Check sheet for the modelled part. Datum: model origin and axes. Units: mm. Face numbers are marked on the shaded views. Give positions to 0.01 mm unless a question says otherwise; leave off trailing zeros. Order: outer loops, then holes, each group sorted by start corner. A loop starts at its lowest first (then second) coordinate and runs counter-clockwise, first axis right, second up.
Autodesk Inventor part; units mm, degrees
ref_plane "YZ Plane" through (0, 0, 0) normal (1, 0, 0) x (0, 1, 0)
ref_plane "XZ Plane" through (0, 0, 0) normal (0, 1, 0) x (-1, 0, 0)
ref_plane "XY Plane" through (0, 0, 0) normal (0, 0, 1) x (1, 0, 0)
sketch "Sketch1" plane through (0, 0, 0) normal (0, 1, 0) x (-1, 0, 0)
  circle A0 centre (0, 0) radius 1.9
  dimension "d0" = 3.8
extrude "Extrusion1" add sketch "Sketch1" along normal blind 6.2
sketch "Sketch2" plane through (0, 6.2, 0) normal (0, 1, 0) x (1, 0, 0)
  line L0 (0, 0) -> (0, -38.1) construction
  line L1 (-4, 0) -> (-4, -38.1)
  line L2 (4, -38.1) -> (4, 0)
  arc A0 (4, 0) -> (-4, 0) centre (0, 0) ccw
  line L3 (4, -38.1) -> (-4, -38.1)
  point P0 (0, -19.05)
  dimension "d6" = 4
  dimension "d7" = 38.1
extrude "Extrusion2" add sketch "Sketch2" along normal blind 0.75 and the other way blind 1.25
sketch "Sketch3" plane through (0, 4.95, 0) normal (0, -1, 0) x (1, 0, 0)
  circle A0 centre (0, 30.48) radius 1.5
  circle A1 centre (0, 0) radius 1.9
  dimension "d11" = 3
  dimension "d12" = 30.48
extrude "Extrusion3" cut sketch "Sketch3" against normal blind 1 contours A0
fillet "Fillet1" radius 1 2 edges at (-4, 5.95, 38.1) (4, 5.95, 38.1)
sketch "Sketch4" plane through (0, 0, 0) normal (0, -1, 0) x (1, 0, 0)
  circle A0 centre (0, 0) radius 1.1
  dimension "d18" = 2.2
extrude "Extrusion4" cut sketch "Sketch4" against normal blind 6.8
properties part number "CC-topHand" material "ABS Plastic"
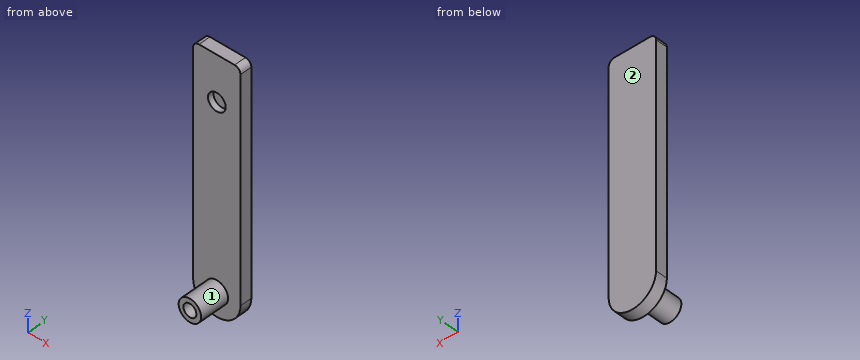
(1) Release check for a two-part mould opening along Z. For the marked faces 1 and 2 record: released by +Z, released by -Z, zero draft, split by the parting line, or undercut.
Response values:
face 1: split by the parting line
face 2: zero draft
(2) Material ranges on L1, parallel to Z at x = 0, y = 5.45; L2, parallel to Y at x = 0.75, z = 4; L3, parallel to X at y = 5.5, z = 1, recorded low to high.
Response values:
L1: z = -4 to -1.1, 1.1 to 28.98, 31.98 to 38.1
L2: y = 4.95 to 6.95
L3: x = -4 to -0.46, 0.46 to 4
(3) Cross-section at C-C on y = 4. Enter the section's corners in (x, z).
Response values:
outline: circle Ø3.8 at (0, 0); hole circle Ø2.2 at (0, 0)
(4) Cross-section at B-B on x = 0. Enter the section's corners in (y, z).
Response values:
outline: (0, -1.9) - (4.95, -1.9) - (4.95, -4) - (6.95, -4) - (6.95, 38.1) - (4.95, 38.1) - (4.95, 31.98) - (5.95, 31.98) - (5.95, 28.98) - (4.95, 28.98) - (4.95, 1.9) - (0, 1.9) - (0, 1.1) - (6.8, 1.1) - (6.8, -1.1) - (0, -1.1) - close
(5) Cross-section at A-A on z = 30.48. Enter the section's corners in (x, y), then the cut area to 3 significant figures.
Response values:
outline: (-4, 4.95) - (-1.5, 4.95) - (-1.5, 5.95) - (1.5, 5.95) - (1.5, 4.95) - (4, 4.95) - (4, 6.95) - (-4, 6.95) - close
area: 13.0 mm2
(6) Gauge pin test, flat ends, axial feed: pin 1 Ø4 at (x, y) = (2, 1) entering from +Z; pin 2 Ø1.5 at (x, z) = (0, 30.5) entering from -Y; pin 3 Ø4 at (x, z) = (1, 21.5) entering from -Y. Record the tip position at first contact, or that the pin passes through.
Response values:
pin 1: stops at z = 1.9
pin 2: stops at y = 5.95
pin 3: stops at y = 4.95
(7) Cross-section at D-D on z = 22. Enter the section's corners in (x, y).
Response values:
outline: (-4, 4.95) - (4, 4.95) - (4, 6.95) - (-4, 6.95) - close
